Input: dimensioned drawing with shaded views. Units: mm. Origin: part minimum x, y, z. Give positions to 0.01 mm unless a question says otherwise; leave off trailing zeros. Order: outer loops, then holes, each group sorted by start corner. A loop starts at its lowest first (then second) coordinate and runs counter-clockwise, first axis right, second up. Notation, with made-up numbers: (-39, -5) - (-26, -5) arc R25 ccw to (-26, 8) - close; hole circle Ø7 at (3.25, 63). An arc over 180 degrees is marked (long way). Use a Markdown table: item, result.
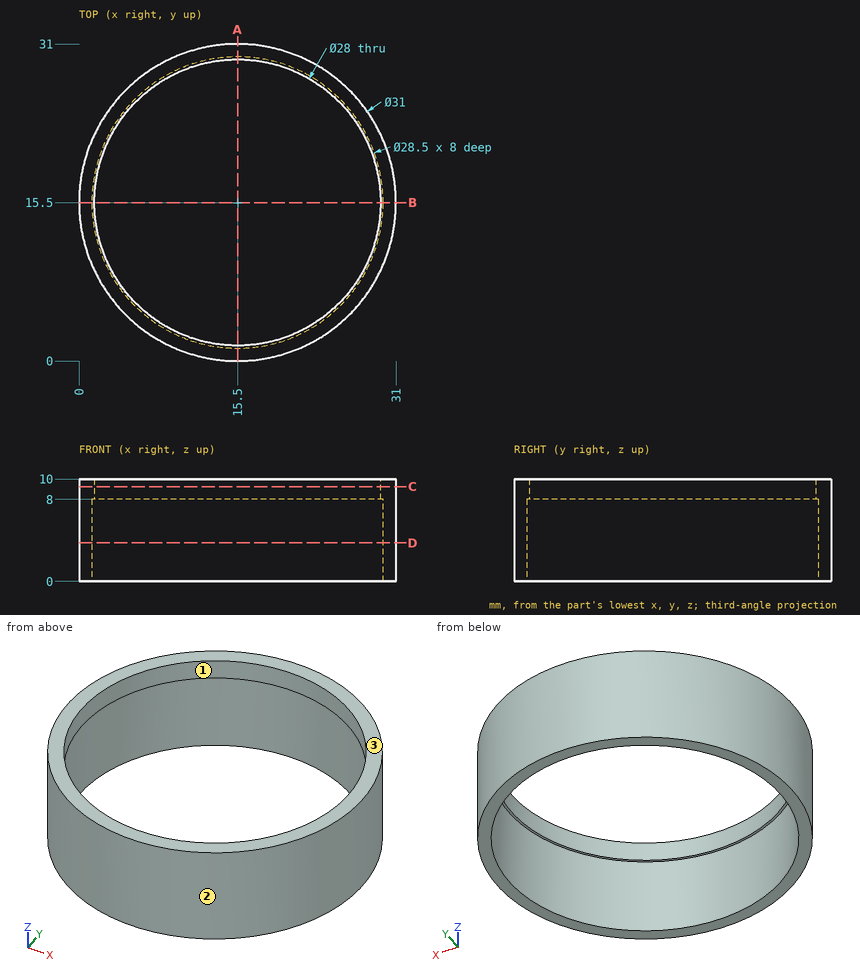
1. Section query A-A (x = 15.5). Return loops of the section in (y, z).
Response:
| item | result |
|---|---|
| outline | (0, 0) - (1.25, 0) - (1.25, 8) - (1.5, 8) - (1.5, 10) - (0, 10) - close; (29.5, 8) - (29.75, 8) - (29.75, 0) - (31, 0) - (31, 10) - (29.5, 10) - close |
2. Pin query (flat end, axial travel): pin 1 (1.5 mm diameter, centred on y = 6, z = 6, fed in from +X); pin 2 (1.5 mm diameter, centred on x = 21, z = 5.5, fed in from +Y); pin 3 (4 mm diameter, centred on x = 24, z = 2.5, fed in from +Y); pin 4 (12 mm diameter, centred on x = 11.5, y = 18.5, fed in from +Z). Return the tip coordinate at first contact, or that it passes through.
Response:
| item | result |
|---|---|
| pin 1 | stops at x = 28.29 |
| pin 2 | stops at y = 30.25 |
| pin 3 | stops at y = 29.57 |
| pin 4 | passes through |
3. Material intervals for line 1 along Y through (x, z) = (15.5, 8.6); line 2 along Y through (x, z) = (15.5, 5.75); line 3 along X through (y, z) = (9, 8.75), sorted ascending.
Response:
| item | result |
|---|---|
| line 1 | y = 0 to 1.5, 29.5 to 31 |
| line 2 | y = 0 to 1.25, 29.75 to 31 |
| line 3 | x = 1.43 to 3.1, 27.9 to 29.57 |
4. Section query D-D (z = 3.75). Return loops of the section in (x, y).
Response:
| item | result |
|---|---|
| outline | circle Ø31 at (15.5, 15.5); hole circle Ø28.5 at (15.5, 15.5) |
5. Section query C-C (z = 9.25). Return loops of the section in (x, y).
Response:
| item | result |
|---|---|
| outline | circle Ø31 at (15.5, 15.5); hole circle Ø28 at (15.5, 15.5) |
6. Mould query, pull axis Y, two halves, no side actions, for the marked faces 1, 2 and 3. Classes: pulls with the +Y half, pulls with the -Y half, needs draft (parallel to the pull), parting line crosses it, or undercut.
Response:
| item | result |
|---|---|
| face 1 | undercut |
| face 2 | parting line crosses it |
| face 3 | needs draft |
